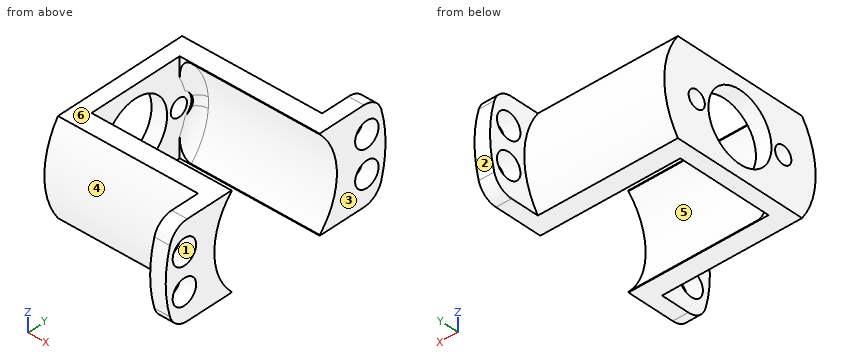
```python
from build123d import *

# Parameters (mm, degrees)
SKETCH2_R               = 3.25
BOSS_EXTRUDE1_DEPTH     = 4
CIRPATTERN2_COUNT       = 2
CUT_EXTRUDE4_DEPTH      = 53.060061468
CUT_EXTRUDE4_DEPTH_BACK = 53.060061468
SKETCH6_W               = 12.790505544
SKETCH6_H               = 56.080299572
SKETCH6_W_2             = 13.13165929
CUT_EXTRUDE5_DEPTH      = 56.733742024
CUT_EXTRUDE5_DEPTH_BACK = 56.733742024
SKETCH8_R               = 2.25
CUT_EXTRUDE6_DEPTH      = 10
FILLET1_R               = 3
SKETCH9_R               = 3.5
CUT_EXTRUDE7_DEPTH      = 30
FILLET2_R               = 5


with BuildPart() as part:
    # Sketch1 → Revolve1 (revolve)
    with BuildSketch(Plane.XY, mode=Mode.PRIVATE) as revolve1_sk:
        Polygon((0, 8.75), (0, 21), (36, 21), (36, 22), (40, 22), (40, 17), (4, 17), (4, 8.75), align=None)
    revolve(revolve1_sk.sketch.rotate(Axis((0, 0, 0), (1, 0, 0)), 90), axis=Axis((0, 0, 0), (1, 0, 0)))

    # Sketch2 → Boss-Extrude1 (add)
    with BuildSketch(Plane(origin=(40, 0, 0), x_dir=(0, 0, -1), z_dir=(1, 0, 0))):
        with BuildLine():
            Line((12, 28.040149786), (12, 18.439088915))
            ThreePointArc((12, 18.439088915), (0, 22), (-12, 18.439088915))
            Line((-12, 18.439088915), (-12, 28.040149786))
            ThreePointArc((-12, 28.040149786), (0, 30.5), (12, 28.040149786))
        make_face()
        with Locations((-4.692554767, 25.318815726)):
            Circle(SKETCH2_R, mode=Mode.SUBTRACT)
        with Locations((4.692554767, 25.318815726)):
            Circle(SKETCH2_R, mode=Mode.SUBTRACT)
    boss_extrude1 = extrude(amount=-BOSS_EXTRUDE1_DEPTH)

    # CirPattern2: Boss-Extrude1 ×2 about axis
    cirpattern2_axis = Axis((0, 0, 0), (1, 0, 0))
    for i in range(1, CIRPATTERN2_COUNT):
        add(boss_extrude1.rotate(cirpattern2_axis, i * 360 / CIRPATTERN2_COUNT))

    # Sketch6 → Cut-Extrude4 (cut, two sides: drawn at the far end of the back side and taken through both)
    with BuildSketch(Plane.ZY.offset(-36).offset(-CUT_EXTRUDE4_DEPTH_BACK)):
        with Locations((-18.395252772, 0)):
            Rectangle(SKETCH6_W, SKETCH6_H)
        with Locations((18.565829645, 0)):
            Rectangle(SKETCH6_W_2, SKETCH6_H)
    extrude(amount=CUT_EXTRUDE4_DEPTH + CUT_EXTRUDE4_DEPTH_BACK, mode=Mode.SUBTRACT)

    # Sketch7 → Cut-Extrude5 (cut, two sides: drawn at the far end of the back side and taken through both)
    with BuildSketch(Plane.XY.offset(12).offset(-CUT_EXTRUDE5_DEPTH_BACK)):
        Polygon((40, 0), (40, 12.23368794), (4, 12.23368794), (4, -12.23368794), (40, -12.23368794), align=None)
    extrude(amount=CUT_EXTRUDE5_DEPTH + CUT_EXTRUDE5_DEPTH_BACK, mode=Mode.SUBTRACT)

    # Sketch8 → Cut-Extrude6 (cut)
    with BuildSketch(Plane.ZY):
        with Locations((0, -12)):
            Circle(SKETCH8_R)
        with Locations((0, 12)):
            Circle(SKETCH8_R)
    extrude(amount=-CUT_EXTRUDE6_DEPTH, mode=Mode.SUBTRACT)

    # Fillet1
    fillet1_edges = [part.edges().sort_by_distance(p)[0] for p in [
        (4, -17, 0),
        (4, 17, 0),
    ]]
    fillet(fillet1_edges, radius=FILLET1_R)

    # Sketch9 → Cut-Extrude7 (cut)
    with BuildSketch(Plane(origin=(4, 0, 0), x_dir=(0, 0, -1), z_dir=(1, 0, 0))):
        with Locations((0, 12)):
            Circle(SKETCH9_R)
        with Locations((0, -12)):
            Circle(SKETCH9_R)
    extrude(amount=CUT_EXTRUDE7_DEPTH, mode=Mode.SUBTRACT)

    # Fillet2
    fillet2_edges = [part.edges().sort_by_distance(p)[0] for p in [
        (38, 28.040149786, -12),
        (38, 28.040149786, 12),
        (38, -28.040149786, 12),
        (38, -28.040149786, -12),
    ]]
    fillet(fillet2_edges, radius=FILLET2_R)


solid = part.part
```
Verification items for the finished model (mm, model axes). Face numbers are marked on the shaded views. A direction names the side the tool comes from. Round coordinates to 2 decimals unless told otherwise and drop trailing zeros. Write each loop counter-clockwise with the first axis right and the second up, starting at its lowest first coordinate (ties: lowest second). Pieces come first, ordered by that corner, then holes.
1. Draft check along Z on the marked faces 1, 2 and 3. Enter one of: +Z half, -Z half, draft (parallel to the pull), parting line (faces both ways), or undercut.
2. Section check A-A on x = 10. Enter the section's corners in (y, z).
3. Section check D-D on y = 20. Enter the section's corners in (x, z), plus the area to 3 significant figures.
4. Gauge pin test, flat ends, axial feed: P1, Ø6.5, axis at y = 22.5, z = 2.5, coming from the -X side; P2, Ø6, axis at x = 22.5, z = 1.5, coming from the -Y side; P3, Ø1.6, axis at x = 16, z = -8.5, coming from the -Y side; P4, Ø1.5, axis at y = -8, z = 1.5, coming from the +X side. Record the tip position at first contact, or that the pin passes through.
5. Section check B-B on x = 37.5. Enter the section's corners in (y, z), plus the area to 3 significant figures.
6. Access from +Z, -Z, +X, -X, +Y, -Y to the whole of each face (thin tool, end or side, straight path). Record for the marked faces 4, 5 and 6.
7. Scan lines: L1, parallel to Y at x = 3.15, z = 0; L2, parallel to X at y = 4, z = 11; L3, parallel to Z at x = 3, y = 12. Record each from-to range of solid material in increasing order.
8. Section check C-C on z = 0. State how many separate pieces and enclosed holes the cut face has, plus the area to 3 significant figures.
Answer:
1. face 1: undercut
1. face 2: parting line
1. face 3: draft
2. outline: (-17.23, -12) - (-12.23, -12) - (-12.23, -11.8) arc R17 cw to (-12.23, 11.8) - (-12.23, 12) - (-17.23, 12) arc R21 ccw to start; (12.23, -12) - (17.23, -12) arc R21 ccw to (17.23, 12) - (12.23, 12) - (12.23, 11.8) arc R17 cw to (12.23, -11.8) - close
3. outline: (0, -6.4) - (36, -6.4) - (36, -12) - (40, -12) - (40, 12) - (36, 12) - (36, 6.4) - (0, 6.4) - close
3. area: 557 mm2
4. P1: stops at x = 0
4. P2: stops at y = -21
4. P3: stops at y = -19.54
4. P4: stops at x = 4
5. outline: (-29.33, -8.37) arc R5 ccw to (-24.52, -12) - (-12.23, -12) - (-12.23, -11.8) arc R17 cw to (-12.23, 11.8) - (-12.23, 12) - (-24.52, 12) arc R5 ccw to (-29.33, 8.37) arc R30.5 ccw to start; (12.23, -12) - (24.52, -12) arc R5 ccw to (29.33, -8.37) arc R30.5 ccw to (29.33, 8.37) arc R5 ccw to (24.52, 12) - (12.23, 12) - (12.23, 11.8) arc R17 cw to (12.23, -11.8) - close; hole circle Ø6.5 at (-25.32, -4.69); hole circle Ø6.5 at (-25.32, 4.69); hole circle Ø6.5 at (25.32, -4.69); hole circle Ø6.5 at (25.32, 4.69)
5. area: 541 mm2
6. face 4: -X, -Y
6. face 5: +X
6. face 6: +Z, +X, -X, +Y, -Y
7. L1: y = -21 to -14.25, -9.75 to -8.75, 8.75 to 9.75, 14.25 to 21
7. L2: x = 0 to 4
7. L3: z = -12 to -2.25, 2.25 to 12
8. separate pieces: 4
8. enclosed holes: 0
8. area: 429 mm2
